from build123d import *

# Parameters (mm, degrees)
SKETCH_W     = 182
SKETCH_H     = 112.2
PAD_DEPTH    = 11
POCKET_DEPTH = 5
FILLET_R     = 7


with BuildPart() as part:
    # Sketch → Pad (new body)
    with BuildSketch(Plane.XY):
        with Locations((91, 56.1)):
            Rectangle(SKETCH_W, SKETCH_H)
    extrude(amount=PAD_DEPTH)

    # Sketch001 (on Face6 of Pad) → Pocket (cut)
    with BuildSketch(Plane.XY.offset(11)):
        with BuildLine():
            ThreePointArc((75, 77.7), (73.5, 79.2), (72, 77.7))
            Line((72, 77.7), (72, 71.798076))
            ThreePointArc((72, 71.798076), (73.5, 66.2), (75, 71.798076))
            Line((75, 71.798076), (75, 77.7))
        make_face()
        with BuildLine():
            ThreePointArc((110, 77.7), (108.5, 79.2), (107, 77.7))
            Line((107, 77.7), (107, 71.798076))
            ThreePointArc((107, 71.798076), (108.5, 66.2), (110, 71.798076))
            Line((110, 71.798076), (110, 77.7))
        make_face()
    extrude(amount=-POCKET_DEPTH, mode=Mode.SUBTRACT)

    # Fillet
    fillet_edges = [part.edges().sort_by_distance(p)[0] for p in [
        (0, 0, 5.5),
        (182, 0, 5.5),
        (182, 112.2, 5.5),
        (0, 112.2, 5.5),
    ]]
    fillet(fillet_edges, radius=FILLET_R)


solid = part.part
Check sheet for the modelled part. Datum: model origin and axes. Units: mm. A direction names the side the tool comes from. Give positions to 0.01 mm unless a question says otherwise; leave off trailing zeros. Loops run counter-clockwise (first coordinate to the right, second up) from the corner with the lowest first, then second, coordinate; pieces in that order, holes last. Notation, with made-up numbers: M 22.25,25.5 L 33.25,25.5 A32 ccw 33.25,62.5 Z; hole C 86,-32 d5. An arc over 180 degrees is marked long. Answer as a JSON object with one key per item and string values. Group by question number.
Q1. Cross-section at A-A on y = 69.2. Record the cut outline in (x, z), then the cut area to 3 significant figures.
Q2. Go/stop test with a flat-tipped pin: P1, Ø3.5, axis at x = 73.5, y = 69.2, coming from the +Z side. Record where the tip stops, or that it passes through.
Q3. Access from +Z, -Z, +X, -X, +Y, -Y to the whole of each face (thin tool, end or side, straight path). Record for faces 5 (the cylindrical face through (2, 110.1, 5.6)), 6 (the flat face through (110, 75, 9)).
Q4. Release check for a two-part mould opening along Y. For faces 1 (the cylindrical face through (2, 2.1, 5.6)), 2 (the flat face through (107, 75, 9)), 3 (the cylindrical face through (179.9, 110.2, 5.6)), 4 (the flat face through (90, 57, 0)) record: released by +Y, released by -Y, zero draft, split by the parting line, or undercut.
Q5. Material ranges on line 1 along X through (y, z) = (69.2, 9); line 2 along Y through (x, z) = (73.5, 7.4), recorded low to high. Write a range as [from, to].
Evaluation:
{
 "1": {"outline": "M 0,0 L 182,0 L 182,11 L 111.5,11 L 111.5,6 L 105.5,6 L 105.5,11 L 76.5,11 L 76.5,6 L 70.5,6 L 70.5,11 L 0,11 Z", "area": "1,940 mm2"},
 "2": {"P1": "stops at z = 6"},
 "3": {"face 5": "+Z, -Z, -X, +Y", "face 6": "+Z"},
 "4": {"face 1": "released by -Y", "face 2": "undercut", "face 3": "released by +Y", "face 4": "zero draft"},
 "5": {"line 1": "x = [0, 70.5], [76.5, 105.5], [111.5, 182]", "line 2": "y = [0, 66.2], [79.2, 112.2]"}
}
